Can you work these out from the drawing? Everything is in mm from the part's minimum corner. A direction names the side the tool comes from. Round coordinates to 2 decimals unless told otherwise and drop trailing zeros. Loops run counter-clockwise (first coordinate to the right, second up) from the corner with the lowest first, then second, coordinate; pieces in that order, holes last. Notation, with made-up numbers: M -8.5,22 L -3.5,22 A18 ccw -3.5,32 Z; hole C 50,4.25 d9. An arc over 180 degrees is marked long. Return JSON: item names as keys, results as strings. Group by question number.
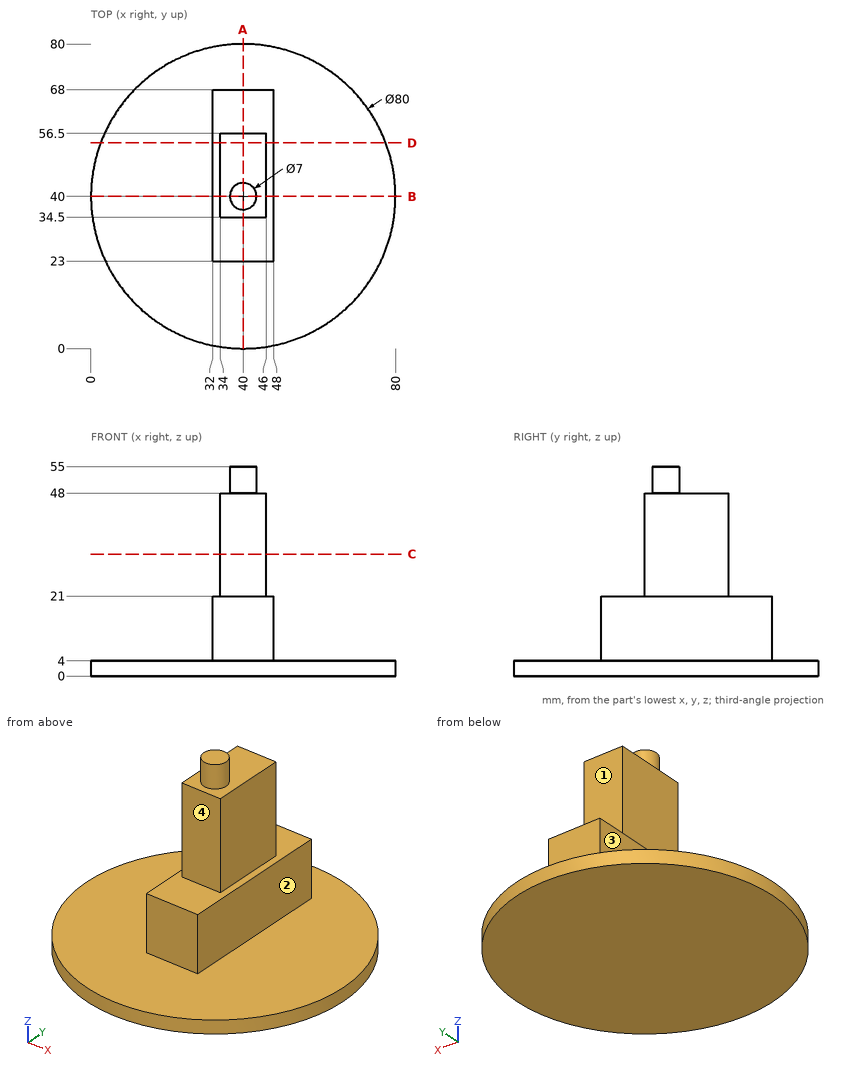
1. I'm going to push flat-ended pins straight in: pin 1 Ø3 at (x, z) = (40.5, 48.5) entering from -Y; pin 2 Ø1 at (x, y) = (29, 41) entering from +Z; pin 3 Ø6.5 at (y, z) = (46, 40) entering from +X; pin 4 Ø3 at (y, z) = (59, 32.5) entering from -X. Where does each tip first touch, or does it pass through?
2. If we section it at D-D, the plane y = 54: Please give me the cut outline in (x, z).
3. On a 3-axis mill with a long thin cutter (end or side, diameter ignored), from which of +Z, -Z, +X, -X, +Y, -Y can I reach the whole of each face in a straight line? I mean the marked faces 1, 2, 3 and 4. Say none if no direction works.
4. If we section it at B-B, the plane y = 40: Please give me the cut outline in (x, z), then the cut area to 3 significant figures.
5. If we section it at C-C, the plane z = 32: Please give me the cut outline in (x, y).
6. I need wall thicknesses on probe 1 along Z at (x, y) = (54, 9.5); probe 2 along X at (y, z) = (37, 40); probe 3 along X at (y, z) = (57.5, 19.5). Which ranges of each line are inside material? Lowest first, please.
7. If we section it at A-A, the plane x = 40: Please give me the cut outline in (y, z).
Geometry results:
{
 "1": {"pin 1": "y = 34.5", "pin 2": "z = 4", "pin 3": "x = 46", "pin 4": "through"},
 "2": {"outline": "M 2.53,0 L 77.47,0 L 77.47,4 L 48,4 L 48,21 L 46,21 L 46,48 L 34,48 L 34,21 L 32,21 L 32,4 L 2.53,4 Z"},
 "3": {"face 1": "+Z, +X, -X, +Y", "face 2": "+Z, +X, +Y, -Y", "face 3": "+Z, -X, +Y, -Y", "face 4": "+Z, +X, -X, -Y"},
 "4": {"outline": "M 0,0 L 80,0 L 80,4 L 48,4 L 48,21 L 46,21 L 46,48 L 43.5,48 L 43.5,55 L 36.5,55 L 36.5,48 L 34,48 L 34,21 L 32,21 L 32,4 L 0,4 Z", "area": "965 mm^2"},
 "5": {"outline": "M 34,34.5 L 46,34.5 L 46,56.5 L 34,56.5 Z"},
 "6": {"probe 1": "0 to 4", "probe 2": "34 to 46", "probe 3": "32 to 48"},
 "7": {"outline": "M 0,0 L 80,0 L 80,4 L 68,4 L 68,21 L 56.5,21 L 56.5,48 L 43.5,48 L 43.5,55 L 36.5,55 L 36.5,48 L 34.5,48 L 34.5,21 L 23,21 L 23,4 L 0,4 Z"}
}
